Design review of the part built by this model. Coordinates are the model's own, in mm. A direction names the side the tool comes from. Round coordinates to 2 decimals unless told otherwise and drop trailing zeros. Write each loop counter-clockwise with the first axis right and the second up, starting at its lowest first coordinate (ties: lowest second). Pieces come first, ordered by that corner, then holes.
from build123d import *

# Parameters (mm, degrees)
IZIM2_W                     = 140
IZIM2_H                     = 60
Y_KSEKLIK_EKSTR_ZYON2_DEPTH = 30
IZIM3_R                     = 6
Y_KSEKLIK_EKSTR_ZYON3_DEPTH = 50


with BuildPart() as part:
    # Çizim2 → Yükseklik-Ekstrüzyon2 (new body)
    with BuildSketch(Plane.XY):
        with Locations((22.258064516, -0.161290323)):
            Rectangle(IZIM2_W, IZIM2_H)
    extrude(amount=Y_KSEKLIK_EKSTR_ZYON2_DEPTH)

    # Çizim3 → Yükseklik-Ekstrüzyon3 (add)
    with BuildSketch(Plane.XY.offset(30)):
        with Locations((43.342230404, -6.03131378)):
            Circle(IZIM3_R)
    extrude(amount=Y_KSEKLIK_EKSTR_ZYON3_DEPTH)


solid = part.part
1) For line 1 along Z through (x, y) = (17, 10); line 2 along X through (y, z) = (-11.5, 57); line 3 along Y through (x, z) = (39.5, 50.5), list the stretches that pass through material, from the lowest coordinate up.
2) For faces 1 (the face through (37.348, -5.768, 54.65)), 2 (the face through (21, 0, 0)), list the 3-axis set-ups (+Z, -Z, +X, -X, +Y, -Y) from which the entire face can be reached by the end or side of a thin tool; tool diameter is ignored.
3) Add section B-B on x = 57. State the section outline as (y, z) points, and give its area (3 significant figures).
4) For P1, Ø18, axis at x = 31, y = 5.5, coming from the +Z side; P2, Ø10, axis at x = 33, z = 50, coming from the +Y side, all flat-tipped, find the tip position at first contact; note any pin that passes through.
5) Add section A-A on y = -23.5. State the section outline as (x, z) points, and give its area (3 significant figures).
Computed:
1. line 1: z = 0 to 30
1. line 2: x = 40.87 to 45.81
1. line 3: y = -10.64 to -1.42
2. face 1: +Z
2. face 2: -Z, +X, -X, +Y, -Y
3. outline: (-30.16, 0) - (29.84, 0) - (29.84, 30) - (-30.16, 30) - close
3. area: 1,800 mm2
4. P1: stops at z = 30
4. P2: stops at y = -3.3
5. outline: (-47.74, 0) - (92.26, 0) - (92.26, 30) - (-47.74, 30) - close
5. area: 4,200 mm2
